Autodesk Inventor part; units mm, degrees
ref_plane "YZ Plane" through (0, 0, 0) normal (1, 0, 0) x (0, 1, 0)
ref_plane "XZ Plane" through (0, 0, 0) normal (0, 1, 0) x (-1, 0, 0)
ref_plane "XY Plane" through (0, 0, 0) normal (0, 0, 1) x (1, 0, 0)
sketch "Sketch1" plane through (0, 0, 0) normal (0, 0, 1) x (1, 0, 0)
  line L0 (0, 0) -> (44.45, 0)
  line L1 (44.45, 0) -> (44.45, 31.75)
  line L2 (44.45, 31.75) -> (31.75, 31.75)
  line L3 (31.75, 31.75) -> (31.75, 0)
  line L4 (0, 0) -> (0, 31.75)
  line L5 (0, 31.75) -> (12.7, 31.75)
  line L6 (12.7, 31.75) -> (12.7, 0)
  line L7 (63.5, -19.05) -> (44.45, 0)
  line L8 (-19.05, -19.05) -> (0, 0)
  line L9 (-19.05, -19.05) -> (-19.05, -57.15)
  line L10 (-19.05, -57.15) -> (0, -57.15)
  line L11 (0, -57.15) -> (63.5, -57.15)
  line L12 (63.5, -57.15) -> (63.5, -19.05)
  dimension "d0" = 44.45
  dimension "d1" = 31.75
  dimension "d2" = 12.7
  dimension "d3" = 31.75
  dimension "d4" = 12.7
  dimension "d9" = 38.1
extrude "Extrusion1" add sketch "Sketch1" against normal blind 127 contours L0 L7 L12 L11 L10 L9 L8
sketch "Sketch2" plane through (0, 0, 0) normal (0, 0, 1) x (1, 0, 0)
  line L0 (63.5, -57.15) -> (-19.05, -57.15)
  arc A0 (47.625, -38.1) -> (-3.175, -38.1) centre (22.225, -38.1) ccw
  line L1 (-3.175, -38.1) -> (-3.175, -57.15)
  line L2 (47.625, -38.1) -> (47.625, -57.15)
  point P0 (0, 0)
  dimension "d14" = 50.8
extrude "Extrusion2" cut sketch "Sketch2" against normal blind 127
sketch "Sketch3" plane through (0, 0, 0) normal (0, 0, 1) x (1, 0, 0)
  line L0 (0, 0) -> (-19.05, -19.05)
  line L1 (0, 0) -> (0, 31.75)
  line L2 (0, 31.75) -> (12.7, 31.75)
  line L3 (12.7, 31.75) -> (12.7, 0)
  line L4 (44.45, 0) -> (0, 0)
  line L5 (44.45, 0) -> (44.45, 31.75)
  line L6 (44.45, 31.75) -> (31.75, 31.75)
  line L7 (31.75, 31.75) -> (31.75, 0)
  dimension "d17" = 31.75
  dimension "d18" = 12.7
  dimension "d19" = 31.75
  dimension "d20" = 12.7
extrude "Extrusion3" add sketch "Sketch3" against normal blind 127 contours L1 L2 L3 L4
sketch "Sketch4" plane through (0, 0, 0) normal (0, 0, 1) x (1, 0, 0)
  line L0 (12.7, 0) -> (44.45, 0)
  line L1 (44.45, 0) -> (44.45, 31.75)
  line L2 (44.45, 31.75) -> (31.75, 31.75)
  line L3 (31.75, 31.75) -> (31.75, 0)
  point P0 (0, 0)
  dimension "d23" = 31.75
  dimension "d24" = 12.7
extrude "Extrusion4" add sketch "Sketch4" against normal blind 127
sketch "Sketch5" plane through (63.5, -57.15, 0) normal (1, 0, 0) x (0, 0, -1)
  line L0 (107.95, 11.1125) -> (107.95, 57.15)
  line L1 (0, 57.15) -> (127, 57.15)
  line L2 (19.05, 10.2158) -> (19.05, 57.15)
  line L3 (107.95, 57.15) -> (19.05, 57.15)
  line L4 (19.05, 10.2158) -> (19.05, 0)
  line L5 (0, 0) -> (127, 0)
  line L6 (107.95, 11.1125) -> (107.95, 0)
extrude "Extrusion5" cut sketch "Sketch5" against normal blind 127
sketch "Sketch6" plane through (0, 0, 0) normal (0, 0, 1) x (1, 0, 0)
  line L0 (12.7, 31.75) -> (33.3375, 31.75)
  line L1 (31.75, 0) -> (31.75, 31.75)
  line L2 (33.3375, 31.75) -> (31.75, 0)
  line L3 (12.7, 0) -> (31.75, 0)
  line L4 (31.75, 0) -> (12.7, 0)
  line L5 (12.7, 31.75) -> (12.7, 0)
  line L6 (12.7, 0) -> (12.7, 31.75)
  point P0 (0, 0)
extrude "Extrusion6" add sketch "Sketch6" against normal blind 127 contours L0 L1 L3 L5
sketch "Sketch7" plane through (44.45, 0, 0) normal (1, 0, 0) x (0, 0, -1)
  line L0 (0, 31.75) -> (127, 31.75)
  circle A0 centre (12.7, 31.75) radius 12.7
  point P0 (0, 0)
  point P1 (25.4, 31.75)
  dimension "d35" = 25.4
extrude "Extrusion7" add sketch "Sketch7" against normal blind 44.45 contours A0 L0 picked at (10.6191, 40.4828)
sketch "Sketch8" plane through (44.45, 0, -127) normal (1, 0, 0) x (0, 0, -1)
  circle A0 centre (-114.3, 31.75) radius 6.35
  point P0 (-127, 0)
  dimension "d39" = 12.7
extrude "Extrusion8" cut sketch "Sketch8" against normal blind 44.45
sketch "Sketch9" plane through (44.45, 0, -127) normal (1, 0, 0) x (0, 0, -1)
  line L0 (-101.6, 31.75) -> (0, 31.75)
  line L1 (-101.6, 31.75) -> (-101.6, 19.05)
  line L2 (-101.6, 19.05) -> (-25.4, 19.05)
  line L3 (-25.4, 19.05) -> (-25.4, 31.75)
  point P0 (-127, 0)
  dimension "d42" = 12.7
extrude "Extrusion9" cut sketch "Sketch9" against normal through all
sketch "Sketch10" plane through (0, 0, 0) normal (0, 0, 1) x (1, 0, 0)
  line L0 (12.7, 0) -> (12.7, 44.45)
  line L1 (31.75, 0) -> (31.75, 44.45)
  line L2 (44.45, 44.45) -> (0, 44.45)
  line L3 (12.7, 44.45) -> (31.75, 44.45)
  line L4 (12.7, 0) -> (31.75, 0)
  line L5 (0, 0) -> (44.45, 0)
  dimension "d50" = 19.05
extrude "Extrusion10" cut sketch "Sketch10" against normal blind 127
properties part number "Assignment 2.4"
For this review, take the finished solid that the model builds, in its own axes (mm). A direction names the side the tool comes from. Round coordinates to 2 decimals unless told otherwise and drop trailing zeros. Write each loop counter-clockwise with the first axis right and the second up, starting at its lowest first coordinate (ties: lowest second). Pieces come first, ordered by that corner, then holes. Notation, with made-up numbers: M 67,65.5 L 84,65.5 A19 cw 84,73.5 Z; hole C 9.25,15.25 d9. An arc over 180 degrees is marked long. Write item = value, one per line. Start each with the question number.
(1) For faces 1 (the face through (38, 31.75, -114)), 2 (the face through (38, 0, -63)), 3 (the face through (38, 25, -25.4)), list the 3-axis set-ups (+Z, -Z, +X, -X, +Y, -Y) from which the entire face can be reached by the end or side of a thin tool; tool diameter is ignored.
(2) We need section B-B (z = -12.7). Give the boundary of the cut face in (x, y) (3 decimals), then the cut area to 3 significant figures.
(3) We need section C-C (x = -11.5). Give the boundary of the cut face in (y, z), then the cut area to 3 significant figures.
(4) For line 1 along Z through (x, y) = (4, -15); line 2 along X through (y, z) = (19, -114.5); line 3 along Z through (x, y) = (2, 31), list the stretches that pass through material, from the lowest coordinate up.
(5) We need section A-A (y = 15). Give the boundary of the cut face in (x, z), then the cut area to 3 significant figures.
(6) The part is to be moulded in two halves that separate along X. For faces 4 (the face through (38.189, 44.447, -12.979)), 5 (the face through (22, 0, -117)), 6 (the face through (-3.175, -47, -9)), 7 (the face through (63.5, -38, -117)), say which applies: +X half, -X half, draft (parallel to the pull), parting line (faces both ways), or undercut.
(7) Clearance check with flat-ended pins moving along their axes: pin 1 Ø5 at (y, z) = (20.5, -79.5) entering from +X; pin 2 Ø10 at (x, z) = (37.5, -49) entering from +Y; pin 3 Ø11.5 at (y, z) = (31.75, -12.7) entering from +X; pin 4 Ø10 at (x, z) = (38, -71.5) entering from -Y. State where each tip first meets the part, or that it passes through.
(8) We need section D-D (y = -25). Give the boundary of the cut face in (x, z).
Results found:
q1.face_1 = -Z, +X, -X, +Y
q1.face_2 = +X, -X, -Y
q1.face_3 = +X, -X, +Y
q2.outline = M -19.05,-57.15 L -3.175,-57.15 L -3.175,-38.1 A25.4 cw 47.625,-38.1 L 47.625,-57.15 L 63.5,-57.15 L 63.5,-19.05 L 44.45,0 L 44.45,25.4 L 31.75,25.4 L 31.75,0 L 12.7,0 L 12.7,25.4 L 0,25.4 L 0,0 L -19.05,-19.05 Z; M 0,38.1 L 12.7,38.1 L 12.7,44.45 L 0,44.45 Z; M 31.75,38.1 L 44.45,38.1 L 44.45,44.45 L 31.75,44.45 Z
q2.area = 3,180 mm²
q3.outline = M -57.15,-127 L -11.5,-127 L -11.5,-107.95 L -57.15,-107.95 Z; M -57.15,-19.05 L -11.5,-19.05 L -11.5,0 L -57.15,0 Z
q3.area = 1,740 mm²
q4.line_1 = -127 to -107.95, -19.05 to 0
q4.line_2 = 0 to 12.7, 31.75 to 44.45
q4.line_3 = -127 to -101.6, -25.4 to -19.01, -6.39 to 0
q5.outline = M 0,-127 L 12.7,-127 L 12.7,0 L 0,0 Z; M 31.75,-127 L 44.45,-127 L 44.45,0 L 31.75,0 Z
q5.area = 3,230 mm²
q6.face_4 = draft
q6.face_5 = undercut
q6.face_6 = undercut
q6.face_7 = +X half
q7.pin_1 = 44.45
q7.pin_2 = 19.05
q7.pin_3 = through
q7.pin_4 = 0
q8.outline = M -19.05,-127 L 0.46,-127 L 0.46,-107.95 L -19.05,-107.95 Z; M -19.05,-19.05 L 0.46,-19.05 L 0.46,0 L -19.05,0 Z; M 43.99,-127 L 63.5,-127 L 63.5,-107.95 L 43.99,-107.95 Z; M 43.99,-19.05 L 63.5,-19.05 L 63.5,0 L 43.99,0 Z
